Can you work these out from the drawing? Everything is in mm from the part's minimum corner. A direction names the side the tool comes from. Give positions to 0.01 mm unless a question says otherwise; leave off trailing zeros. Order: outer loops, then holes, each group sorted by start corner. A loop starts at its lowest first (then second) coordinate and runs counter-clockwise, first axis right, second up. Notation, with made-up numbers: (4.25, 60) - (22.25, 60) arc R4 cw to (22.25, 67) - close; hole circle Ø7 at (31, 47). An arc over 180 degrees is marked (long way). One line per question, with ' | ' between items.
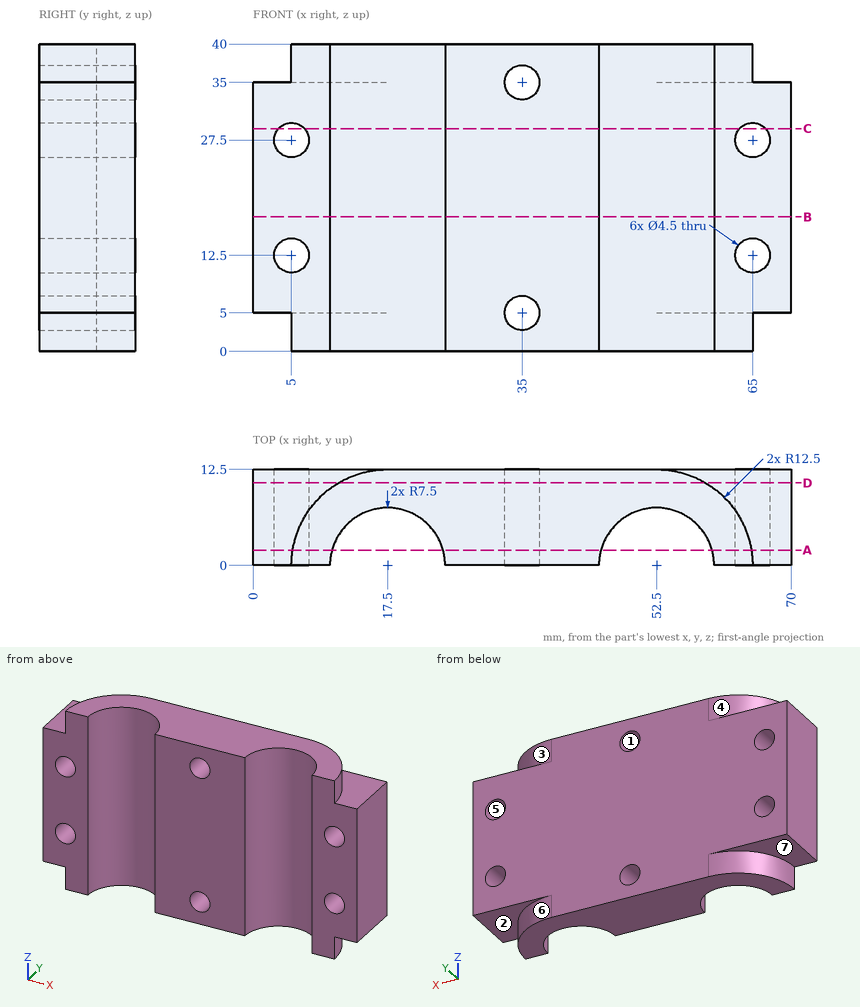
(1) Imagine slicing it at C-C (z = 29). List the corners of the cut face in (x, y) for me, and give its area (3 significant figures).
Answer below:
outline: (0, 0) - (3.32, 0) - (3.32, 12.5) - (0, 12.5) - close; (6.68, 0) - (10, 0) arc R7.5 cw to (25, 0) - (45, 0) arc R7.5 cw to (60, 0) - (63.32, 0) - (63.32, 12.5) - (6.68, 12.5) - close; (66.68, 0) - (70, 0) - (70, 12.5) - (66.68, 12.5) - close | area: 614 mm^2
(2) If we mould it in two halves opening along X, with no side actions, what happens to the marked faces 5, 6 and 7? For each: released by +X, released by -X, zero draft, split by the parting line, or undercut.
Answer below:
face 5: undercut | face 6: released by +X | face 7: zero draft
(3) On a 3-axis mill with a long thin cutter (end or side, diameter ignored), from which of +Z, -Z, +X, -X, +Y, -Y can I reach the whole of each face in a straight line? I mean the marked faces 1, 2, 3 and 4. Say none if no direction works.
Answer below:
face 1: +Y, -Y | face 2: -Z, +X, +Y | face 3: +Z, +X, +Y | face 4: +Z, -X, +Y
(4) If I drill on line 1 (Z direction, x = 65, y = 4); line 2 (X direction, y = 8.25, z = 25.5); line 3 (X direction, y = 6, z = 33), over which ranges is the centre line in solid material (lowest first)?
Answer below:
line 1: 5 to 10.25, 14.75 to 25.25, 29.75 to 35 | line 2: 0 to 3.97, 6.03 to 63.97, 66.03 to 70 | line 3: 0 to 13, 22 to 33.97, 36.03 to 48, 57 to 70
(5) Imagine slicing it at D-D (y = 10.75). List the corners of the cut face in (x, z) for me, and give its area (3 significant figures).
Answer below:
outline: (0, 5) - (11.12, 5) - (11.12, 0) - (58.88, 0) - (58.88, 5) - (70, 5) - (70, 35) - (58.88, 35) - (58.88, 40) - (11.12, 40) - (11.12, 35) - (0, 35) - close; hole circle Ø4.5 at (5, 12.5); hole circle Ø4.5 at (5, 27.5); hole circle Ø4.5 at (35, 5); hole circle Ø4.5 at (35, 35); hole circle Ø4.5 at (65, 12.5); hole circle Ø4.5 at (65, 27.5) | area: 2,480 mm^2
(6) Imagine slicing it at A-A (y = 2). Count the separate pieces of the cut face and the enclosed holes in it, and give its area (3 significant figures).
Answer below:
separate pieces: 3 | enclosed holes: 6 | area: 1,440 mm^2
(7) Imagine slicing it at B-B (z = 17.5). List the corners of the cut face in (x, y) for me.
Answer below:
outline: (0, 0) - (10, 0) arc R7.5 cw to (25, 0) - (45, 0) arc R7.5 cw to (60, 0) - (70, 0) - (70, 12.5) - (0, 12.5) - close
(8) Will these pins go through, and if not, where does the flat tip stop? pin 1 (2 mm diameter, centred on x = 47, y = 10.5, fed in from -Z); pin 2 (4 mm diameter, centred on x = 65, z = 27.5, fed in from -Y).
Answer below:
pin 1: z = 0 | pin 2: through
